Autodesk Inventor part; units mm, degrees
ref_plane "YZ Plane" through (0, 0, 0) normal (1, 0, 0) x (0, 1, 0)
ref_plane "XZ Plane" through (0, 0, 0) normal (0, 1, 0) x (-1, 0, 0)
ref_plane "XY Plane" through (0, 0, 0) normal (0, 0, 1) x (1, 0, 0)
sketch "Sketch1" plane through (0, 0, 0) normal (0, 1, 0) x (-1, 0, 0)
  line L0 (0, 0) -> (100, 0)
  line L1 (100, 0) -> (100, -100)
  line L2 (100, -100) -> (0, -100)
  line L3 (0, -100) -> (0, 0)
  line L4 (100, -50) -> (0, -50) construction
  line L5 (7.1, -7.5) -> (92.9, -7.5) construction
  line L6 (92.9, -7.5) -> (92.9, -92.5) construction
  line L7 (92.9, -92.5) -> (7.1, -92.5) construction
  line L8 (7.1, -92.5) -> (7.1, -7.5) construction
  line L9 (7.1, -7.5) -> (92.9, -92.5) construction
  line L10 (92.9, -7.5) -> (7.1, -92.5) construction
  circle A0 centre (92.9, -7.5) radius 1.5
  circle A1 centre (92.9, -92.5) radius 1.5
  circle A2 centre (7.1, -92.5) radius 1.5
  circle A3 centre (7.1, -7.5) radius 1.5
  point P0 (50, -50)
  dimension "d0" = 100
  dimension "d1" = 100
  dimension "d2" = 85.8
  dimension "d3" = 85
  dimension "d4" = 3
  dimension "d5" = 3
  dimension "d6" = 3
  dimension "d7" = 3
extrude "Extrusion1" add sketch "Sketch1" along normal blind 5
sketch "Sketch2" plane through (0, 5, 0) normal (0, 1, 0) x (1, 0, 0)
  line L0 (-100, 100) -> (-100, 0)
  line L1 (-100, 30) -> (-97, 30)
  line L2 (-97, 30) -> (-97, 70)
  line L3 (-97, 70) -> (-100, 70)
  line L4 (-100, 70) -> (-100, 30)
  line L5 (-97, 50) -> (-100, 50) construction
  line L6 (0, 0) -> (0, 100)
  line L7 (0, 50) -> (-100, 50) construction
  line L8 (-100, 0) -> (0, 0)
  line L9 (-50, 0) -> (-50, 98) construction
  line L10 (-70, 0) -> (-30, 0)
  line L11 (-30, 0) -> (-30, 3)
  line L12 (-30, 3) -> (-70, 3)
  line L13 (-70, 3) -> (-70, 0)
  line L14 (-50, 3) -> (-50, 0) construction
  line L15 (0, 30) -> (-3, 30)
  line L16 (-3, 30) -> (-3, 70)
  line L17 (-3, 70) -> (0, 70)
  line L18 (0, 70) -> (0, 30)
  line L19 (-3, 50) -> (0, 50) construction
  line L20 (-70, 100) -> (-30, 100)
  line L21 (-30, 100) -> (-30, 97)
  line L22 (-30, 97) -> (-70, 97)
  line L23 (-70, 97) -> (-70, 100)
  line L24 (-50, 97) -> (-50, 100) construction
  dimension "d10" = 40
  dimension "d11" = 3
  dimension "d12" = 40
  dimension "d13" = 3
extrude "Extrusion2" [suppressed]
properties part number "Base"
The model under review builds one solid part; all positions refer to its coordinate system, in mm. Round coordinates to 2 decimals unless told otherwise and drop trailing zeros. Write each loop counter-clockwise with the first axis right and the second up, starting at its lowest first coordinate (ties: lowest second). Pieces come first, ordered by that corner, then holes. Notation, with made-up numbers: (11, 11.25) - (53, 11.25) arc R31 cw to (53, 40.25) - close; hole circle Ø10 at (12.25, 18.5). An arc over 180 degrees is marked (long way). One line per question, with ' | ' between items.
Item 1: The part is to be moulded in two halves that separate along X. For faces 1 (the face through (-49, 5, -49)), 2 (the face through (0, 2, -51)), 3 (the face through (-7.79, 2.46, -6.17)), 4 (the face through (-91.4, 2.46, -7.57)), say which applies: pulls with the +X half, pulls with the -X half, needs draft (parallel to the pull), parting line crosses it, or undercut.
Resolved:
face 1: needs draft | face 2: pulls with the +X half | face 3: undercut | face 4: undercut
Item 2: Add section A-A, the plane z = -92.5. Give the boundary of the cut face in (x, y), then the cut area to 3 significant figures.
Resolved:
outline: (-100, 0) - (-94.4, 0) - (-94.4, 5) - (-100, 5) - close; (-91.4, 0) - (-8.6, 0) - (-8.6, 5) - (-91.4, 5) - close; (-5.6, 0) - (0, 0) - (0, 5) - (-5.6, 5) - close | area: 470 mm2
Item 3: To check wall thickness, follow probe 1 along X at (y, z) = (3.85, -92.5); probe 2 along Z at (x, y) = (-7.1, 2.3). State the ranges of each line that lie inside material, in increasing order.
Resolved:
probe 1: x = -100 to -94.4, -91.4 to -8.6, -5.6 to 0 | probe 2: z = -100 to -94, -91 to -9, -6 to 0
Item 4: Add section B-B, the plane x = -7.1. Give the boundary of the cut face in (y, z), then the cut area to 3 significant figures.
Resolved:
outline: (0, -100) - (5, -100) - (5, -94) - (0, -94) - close; (0, -91) - (5, -91) - (5, -9) - (0, -9) - close; (0, -6) - (5, -6) - (5, 0) - (0, 0) - close | area: 470 mm2
